Part model, mm, in its own coordinate system. A direction names the side the tool comes from. Round coordinates to 2 decimals unless told otherwise and drop trailing zeros. Order: outer loops, then holes, each group sorted by start corner. A loop starts at its lowest first (then second) coordinate and runs counter-clockwise, first axis right, second up. Notation, with made-up numbers: (78.5, -14.75) - (126.5, -14.75) arc R28 ccw to (126.5, 7.25) - close; hole circle Ø11 at (54.25, 57). An arc over 180 degrees is marked (long way). Return JSON: item names as keys, results as strings. Group by question number.
Item 1: Saw through at B-B on x = 0. List the corners of the cut face in (y, z).
Item 2: Two-plate mould, pull along Y, no slides. Class faces 1 (the face through (91.074, 46.838, 4.93)), 2 (the face through (36, 36, 10)), 3 (the face through (0, -1.588, 5)): released by +Y, released by -Y, zero draft, split by the parting line, or undercut.
Item 3: Saw through at C-C on y = 0. List the corners of the cut face in (x, z).
Item 4: Drop flat-ended pins along their axis: pin 1 (1 mm diameter, centred on x = 86, z = 3.5, fed in from +Y); pin 2 (3 mm diameter, centred on y = 27, z = 9, fed in from +X); pin 3 (1.6 mm diameter, centred on x = 0.5, z = 5, fed in from -Y); pin 4 (3.5 mm diameter, centred on x = 86, z = 6.5, fed in from -Y). Give the stop position or say it passes through.
Item 5: Probe probe 1 along X at (y, z) = (48, 7.25); probe 2 along Y at (x, z) = (72, 8.5); probe 3 along Y at (x, z) = (1, 8.5). List the from-to ranges inside material, lowest first.
Item 6: Saw through at D-D on y = 41.5. List the corners of the cut face in (x, z).
Item 7: Saw through at A-A on z = 2.5. List the corners of the cut face in (x, y), and give its area (3 significant figures).
Item 8: Tool access for faces 4 (the face through (1.588, 0, 5)), 5 (the face through (36.247, 34.743, 4.93)): list every direction of +Z, -Z, +X, -X, +Y, -Y with a clear straight run to the whole face (end or side of a thin tool).
```python
from build123d import *

# Parameters (mm, degrees)
SKETCH1_W           = 3.175
SKETCH1_H           = 3.175
BOSS_EXTRUDE1_DEPTH = 10


with BuildPart() as part:
    # Sketch1 → Boss-Extrude1 (new body)
    with BuildSketch(Plane.XY):
        with BuildLine():
            ThreePointArc((87.048054742, 52.882382784), (31.917584067, 43.964642964), (-4.738476051, 1.831186697))
            ThreePointArc((-4.738476051, 1.831186697), (-1.831186697, -4.738476051), (4.738476051, -1.831186697))
            ThreePointArc((4.738476051, -1.831186697), (36.856053246, 35.085615868), (85.160675784, 42.899226937))
            ThreePointArc((85.160675784, 42.899226937), (91.095943187, 46.947115382), (87.048054742, 52.882382784))
        make_face()
        Rectangle(SKETCH1_W, SKETCH1_H, mode=Mode.SUBTRACT)
        with Locations((86.104365263, 47.890804861)):
            Rectangle(SKETCH1_W, SKETCH1_H, mode=Mode.SUBTRACT)
    extrude(amount=BOSS_EXTRUDE1_DEPTH)


solid = part.part
```
Filled in:
{
 "1": {"outline": "(-5.08, 0) - (-1.59, 0) - (-1.59, 10) - (-5.08, 10) - close; (1.59, 0) - (11.97, 0) - (11.97, 10) - (1.59, 10) - close"},
 "2": {"face 1": "split by the parting line", "face 2": "zero draft", "face 3": "undercut"},
 "3": {"outline": "(-5.08, 0) - (-1.59, 0) - (-1.59, 10) - (-5.08, 10) - close; (1.59, 0) - (5.48, 0) - (5.48, 10) - (1.59, 10) - close"},
 "4": {"pin 1": "stops at y = 53.16", "pin 2": "stops at x = 27.02", "pin 3": "stops at y = -5.08", "pin 4": "stops at y = 42.81"},
 "5": {"probe 1": "x = 40.25 to 84.52, 87.69 to 91.18", "probe 2": "y = 44.15 to 54.31", "probe 3": "y = -4.98 to -1.59, 1.59 to 13.73"},
 "6": {"outline": "(27.78, 0) - (52.46, 0) - (52.46, 10) - (27.78, 10) - close"},
 "7": {"outline": "(-4.74, 1.83) arc R5.08 ccw to (4.74, -1.83) arc R71.9 cw to (85.16, 42.9) arc R5.08 ccw to (87.05, 52.88) arc R82.06 ccw to start; hole (-1.59, -1.59) - (1.59, -1.59) - (1.59, 1.59) - (-1.59, 1.59) - close; hole (84.52, 46.3) - (87.69, 46.3) - (87.69, 49.48) - (84.52, 49.48) - close", "area": "1,150 mm^2"},
 "8": {"face 4": "+Z, -Z", "face 5": "+Z, -Z, -Y"}
}
